Autodesk Inventor part; units mm, degrees
ref_plane "YZ Plane" through (0, 0, 0) normal (1, 0, 0) x (0, 1, 0)
ref_plane "XZ Plane" through (0, 0, 0) normal (0, 1, 0) x (-1, 0, 0)
ref_plane "XY Plane" through (0, 0, 0) normal (0, 0, 1) x (1, 0, 0)
sketch "Sketch1" plane through (0, 0, 0) normal (0, 0, 1) x (1, 0, 0)
  line L0 (-12.2838, 5.95) -> (-117.2838, 5.95)
  line L1 (-117.2838, 5.95) -> (-117.2838, -64.05)
  line L2 (-117.2838, -64.05) -> (-12.2838, -64.05)
  line L3 (-12.2838, -64.05) -> (-12.2838, 5.95)
  point P0 (0, 0)
  dimension "d0" = 105
  dimension "d1" = 70
extrude "Extrusion1" add sketch "Sketch1" along normal blind 12
chamfer "Chamfer1" distance 4 angle 45 4 edges at (-12.2838, 5.95, 6) (-12.2838, -64.05, 6) (-117.2838, -64.05, 6) (-117.2838, 5.95, 6)
sketch "Sketch2" plane through (0, 0, 12) normal (0, 0, 1) x (1, 0, 0)
  line L0 (-103.2855, -8.853) -> (-76.1362, -8.853)
  line L1 (-76.1362, -8.853) -> (-76.1362, -50.7574)
  line L2 (-76.1362, -50.7574) -> (-103.2855, -50.7574)
  line L3 (-103.2855, -50.7574) -> (-103.2855, -8.853)
  point P0 (0, 0)
extrude "Extrusion2" cut sketch "Sketch2" against normal blind 3
chamfer "Chamfer2" distance 2 angle 45 4 edges at (-103.2855, -29.8052, 12) (-89.7108, -8.853, 12) (-76.1362, -29.8052, 12) (-89.7108, -50.7574, 12)
properties part number "RFID scanner"
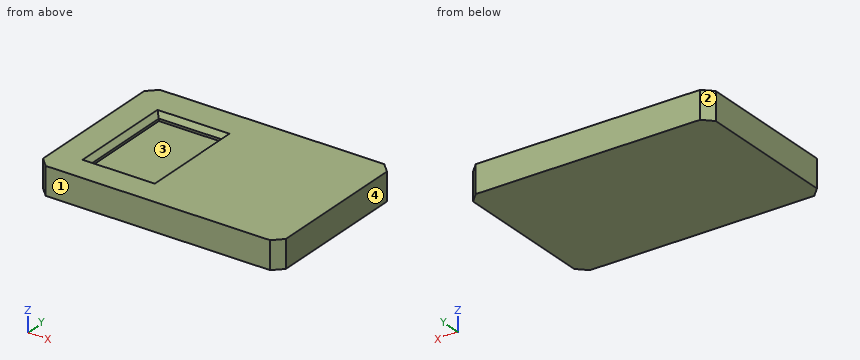
Model file for the job. Use its own axes, mm. Face numbers are marked on the shaded views. Round coordinates to 2 decimals unless told otherwise and drop trailing zeros. Write each loop counter-clockwise with the first axis right and the second up, starting at its lowest first coordinate (ties: lowest second). Pieces come first, ordered by that corner, then holes. Notation, with made-up numbers: M 5.25,24.25 L 42.25,24.25 A34 cw 42.25,58.25 Z; hole C 45.5,-5 d9. An arc over 180 degrees is marked long. Put each result on its own line as item: value.
Item 1: Mould opens along Y. For the marked faces 1, 2, 3 and 4 say: +Y half, -Y half, draft (parallel to the pull), parting line (faces both ways), or undercut.
Responses:
face 1: -Y half
face 2: +Y half
face 3: undercut
face 4: draft
Item 2: Probe L1, parallel to Z at x = -94, y = -42; L2, parallel to X at y = 3.5, z = 5. List the from-to ranges inside material, lowest first. Write a range as from..to.
Responses:
L1: 0..9
L2: -115.73..-13.83
Item 3: Cut at A-A (y = -27). List the corners of the cut face in (x, z).
Responses:
outline: M -117.28,0 L -12.28,0 L -12.28,12 L -74.14,12 L -76.14,10 L -76.14,9 L -103.29,9 L -103.29,10 L -105.29,12 L -117.28,12 Z
Item 4: Flat gauge pin, fed straight in: P1, Ø6, axis at x = -77.5, y = -36.5, coming from the +Z side. Where does the tip first touch, or does it go through?
Responses:
P1: z = 11.64
Item 5: Cut at B-B (x = -101.5). List the corners of the cut face in (y, z), and give its area (3 significant figures).
Responses:
outline: M -64.05,0 L 5.95,0 L 5.95,12 L -6.85,12 L -8.85,10 L -8.85,9 L -50.76,9 L -50.76,10 L -52.76,12 L -64.05,12 Z
area: 710 mm²
